from build123d import *

# Parameters (mm, degrees)
BOSS_EXTRUDE1_DEPTH = 476.25
SKETCH2_R           = 1.984375
CUT_EXTRUDE1_DEPTH  = 477.43707659
SKETCH3_R           = 1.984375
CUT_EXTRUDE2_DEPTH  = 477.43707659
SKETCH4_R           = 1.984375
CUT_EXTRUDE3_DEPTH  = 477.43707659
SKETCH5_R           = 1.984375
CUT_EXTRUDE4_DEPTH  = 477.43707659


with BuildPart() as part:
    # Sketch1 → Boss-Extrude1 (new body)
    with BuildSketch(Plane.XY):
        Polygon((0, 0), (-8.980256121, 8.980256121), (-9.878281733, 8.082230509), (0, -1.796051224), (9.878281733, 8.082230509), (8.980256121, 8.980256121), align=None)
    extrude(amount=BOSS_EXTRUDE1_DEPTH)

    # Sketch2 → Cut-Extrude1 (cut, through all)
    with BuildSketch(Plane(origin=(0, 0, 0), x_dir=(0, 0, 1), z_dir=(-0.7071067811865469, 0.7071067811865481, 0))):
        with Locations(Location((469.9, 6.35, 0), (0, 0, 270))):
            Circle(SKETCH2_R)
        with Locations(Location((457.2, 6.35, 0), (0, 0, 270))):
            Circle(SKETCH2_R)
    extrude(amount=-CUT_EXTRUDE1_DEPTH, mode=Mode.SUBTRACT)

    # Sketch3 → Cut-Extrude2 (cut, through all)
    with BuildSketch(Plane(origin=(0, 0, 0), x_dir=(0, 0, -1), z_dir=(0.7071067811865483, 0.7071067811865468, 0))):
        with Locations(Location((-463.55, 6.35, 0), (0, 0, 90))):
            Circle(SKETCH3_R)
    extrude(amount=-CUT_EXTRUDE2_DEPTH, mode=Mode.SUBTRACT)

    # Sketch4 → Cut-Extrude3 (cut, through all)
    with BuildSketch(Plane(origin=(0, 0, 0), x_dir=(0, 0, 1), z_dir=(-0.7071067811865471, 0.7071067811865479, 0))):
        with Locations(Location((6.35, 6.35, 0), (0, 0, 270))):
            Circle(SKETCH4_R)
        with Locations(Location((19.05, 6.35, 0), (0, 0, 270))):
            Circle(SKETCH4_R)
    extrude(amount=-CUT_EXTRUDE3_DEPTH, mode=Mode.SUBTRACT)

    # Sketch5 → Cut-Extrude4 (cut, through all)
    with BuildSketch(Plane(origin=(0, 0, 0), x_dir=(0, 0, -1), z_dir=(0.7071067811865482, 0.7071067811865468, 0))):
        with Locations(Location((-12.7, 6.35, 0), (0, 0, 90))):
            Circle(SKETCH5_R)
    extrude(amount=-CUT_EXTRUDE4_DEPTH, mode=Mode.SUBTRACT)


solid = part.part
Can you work these out from the model? Positions are in its coordinate system, mm. A direction names the side the tool comes from. Give positions to 0.01 mm unless a question says otherwise; leave off trailing zeros. Loops run counter-clockwise (first coordinate to the right, second up) from the corner with the lowest first, then second, coordinate; pieces in that order, holes last. Notation, with made-up numbers: (22, -6.5) -> (77, -6.5) arc R34 ccw to (77, 31.5) -> close; hole circle Ø9 at (54.5, -12.75). An arc over 180 degrees is marked (long way). Write item = value, one per line.
1) Thinking about a two-plate mould opening in X: for faces 3 (the flat face through (4.87, 3.074, 234.791)), 4 (the flat face through (5, 5, 235)), 5 (the flat face through (-2.24, 2.02, 0)), which applies, released by +X, released by -X, zero draft, split by the parting line, or undercut?
Check result:
face_3 = released by +X
face_4 = undercut
face_5 = zero draft
2) Suppose I cut it at A-A on z = 189. Write out the boundary of the cut face in (x, y), then the cut area to 3 significant figures.
Check result:
outline = (-9.88, 8.08) -> (0, -1.8) -> (9.88, 8.08) -> (8.98, 8.98) -> (0, 0) -> (-8.98, 8.98) -> close
area = 33.9 mm2
3) Will these pins go through, and if not, where does the flat tip stop? pin 1 (6 mm diameter, centred on x = 5, z = 420, fed in from -Y); pin 2 (5 mm diameter, centred on x = -8, z = 401, fed in from -Y); pin 3 (2 mm diameter, centred on x = 2.5, z = 224, fed in from +Y).
Check result:
pin_1 = 0.2
pin_2 = 3.7
pin_3 = 3.5
4) For faces 1 (the flat face through (-4, 4, 235)), 2 (the flat face through (-5.008, 3.212, 234.791)), which set-ups out of +Z, -Z, +X, -X, +Y, -Y let a thin tool reach every point of the face, with its end or its side?
Check result:
face_1 = +Z, -Z, +Y
face_2 = +Z, -Z, -X, -Y
5) I need wall thicknesses on L1, parallel to Z at x = -5.25, y = 3.5; L2, parallel to X at y = 1, z = 337; L3, parallel to X at y = 0.25, z = 158. Which ranges of each line are inside material? Lowest first, please. Write a range as from..to.
Check result:
L1 = 0..10.72, 14.68..461.57, 465.53..476.25
L2 = -2.8..-1, 1..2.8
L3 = -2.05..-0.25, 0.25..2.05
